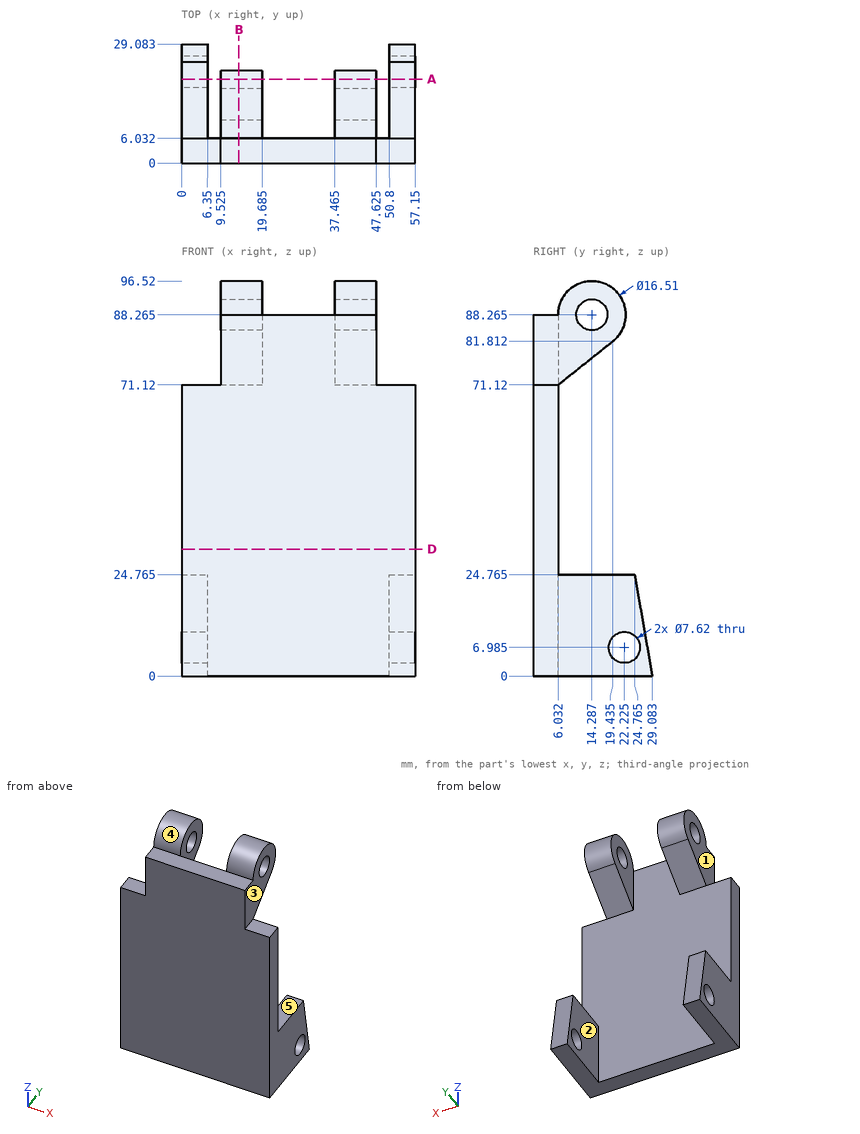
Print and shaded views of the part. All mm, measured from the part's lowest x, y and z. A direction names the side the tool comes from. Round coordinates to 2 decimals unless told otherwise and drop trailing zeros. Write each loop counter-clockwise with the first axis right and the second up, starting at its lowest first coordinate (ties: lowest second). Pieces come first, ordered by that corner, then holes. Notation, with made-up numbers: M 46.5,65 L 71.5,65 A33 cw 71.5,101 Z; hole C -3.5,71 d10. An arc over 180 degrees is marked long. Use a Markdown table: item, result. Add a question column.
1. Slice it at D-D on z = 31. Give the cut face in (x, y).
2. 3-axis set-ups, long thin cutter, end or side, ignore diameter. For the marked faces 1, 2, 3, 4 and 5: which of +Z, -Z, +X, -X, +Y, -Y reach the whole face in a straight line?
3. Flat gauge pins, fed straight in: P1, Ø7, axis at x = 2, y = 14.5, coming from the +Z side (1 decimal); P2, Ø5, axis at x = 19.5, y = 4.5, coming from the +Z side (1 decimal); P3, Ø13, axis at y = 10.5, z = 85.5, coming from the +X side (1 decimal). Where does each tip first touch, or does it go through?
4. Slice it at B-B on x = 14. Give the cut face in (y, z) (1 decimal).
5. Slice it at A-A on y = 20.5. Give the number of separate pieces and of enclosed holes in the cut face, then the cut area to 3 significant figures.
6. Drill centre lines: probe 1 along X at (y, z) = (7, 18.5); probe 2 along Z at (x, y) = (36, 3.5) (1 decimal); probe 3 along Y at (x, z) = (44.5, 40). Where is each one in solid material? Low to high.
Reply:
| question | item | result |
|---|---|---|
| 1 | outline | M 0,0 L 57.15,0 L 57.15,6.03 L 0,6.03 Z |
| 2 | face 1 | +Z, -X, +Y, -Y |
| 2 | face 2 | +Z, -Z, +Y |
| 2 | face 3 | +Z, +X, +Y, -Y |
| 2 | face 4 | +X, -X |
| 2 | face 5 | +Z, +X, -X, +Y |
| 3 | P1 | stops at z = 24.8 |
| 3 | P2 | stops at z = 92.1 |
| 3 | P3 | stops at x = 47.6 |
| 4 | outline | M 0,0 L 6,0 L 6,71.1 L 19.4,81.8 A8.3 ccw long 6,88.3 L 0,88.3 Z; hole C 14.3,88.3 d7.6 |
| 5 | separate pieces | 6 |
| 5 | enclosed holes | 0 |
| 5 | area | 449 mm^2 |
| 6 | probe 1 | x = 0 to 6.35, 50.8 to 57.15 |
| 6 | probe 2 | z = 0 to 88.3 |
| 6 | probe 3 | y = 0 to 6.03 |
